```python
from build123d import *

# Parameters (mm, degrees)
F1_DEPTH = 25.4


with BuildPart() as f1:
    # F0 (on Right) → F1 (new body)
    with BuildSketch(Plane.YZ):
        with BuildLine():
            Line((-304.8, 0), (0, 0))
            Line((0, 0), (31.860275604, 303.1302737082))
            ThreePointArc((31.860275604, 303.1302737082), (-25.6710248369, 296.0445279913), (-65.6702667475, 254.0907561779))
            add(Edge.make_bspline(
                [(-246.146813035, 87.6441970468), (-194.5365692681, 86.4305306387), (-88.5158652272, 83.9373479358), (-73.4183843518, 196.3829828835), (-65.6702667475, 254.0907561779)],
                knots=[0, 0, 0, 0, 0.486794011, 1, 1, 1, 1], degree=3))
            ThreePointArc((-246.146813035, 87.6441970468), (-289.5827369697, 53.2643345738), (-304.8, 0))
        make_face()
    extrude(amount=F1_DEPTH)


solid = f1.part
```
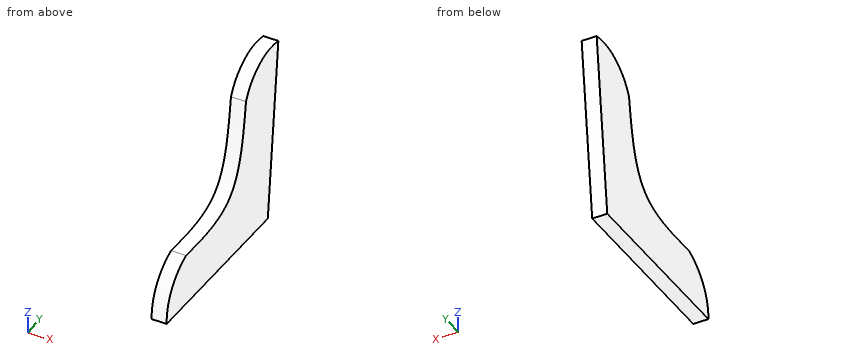
Read the model definition and answer for the solid it produces. Units are mm, in the model's axes. Give positions to 0.01 mm unless a question says otherwise; leave off trailing zeros. Order: outer loops, then holes, each group sorted by start corner. A loop starts at its lowest first (then second) coordinate and runs counter-clockwise, first axis right, second up.
(1) Find section B-B (y = -18). Give the vertices of the cut face in (x, z).
(2) Find section A-A (z = 36.5). Give the vertices of the cut face in (x, y), plus the area to 3 significant figures.
(3) Straight lines are drawn through the part: L1, parallel to Z at x = 13, y = -161; L2, parallel to Z at x = 17.5, y = -122; L3, parallel to Y at x = 14, z = 197.5. For each, find the intervals that lie inside material, in ascending order.
(4) Given pin 1 (10 mm diameter, centred on x = 19.5, y = -23, fed in from +Z); pin 2 (8 mm diameter, centred on x = 5, z = 116.5, fed in from -Y); pin 3 (6 mm diameter, centred on x = 18.5, z = 203.5, fed in from -Y), each flat-ended and moving along its own axis, determine where each tip first touches the part or whether it passes through.
Result sheet:
1. outline: (0, 0) - (25.4, 0) - (25.4, 299.44) - (0, 299.44) - close
2. outline: (0, -298.41) - (25.4, -298.41) - (25.4, 3.84) - (0, 3.84) - close
2. area: 7,680 mm2
3. L1: z = 0 to 90.77
3. L2: z = 0 to 104.53
3. L3: y = -74.31 to 20.76
4. pin 1: stops at z = 299.44
4. pin 2: stops at y = -111.45
4. pin 3: stops at y = -73.74
